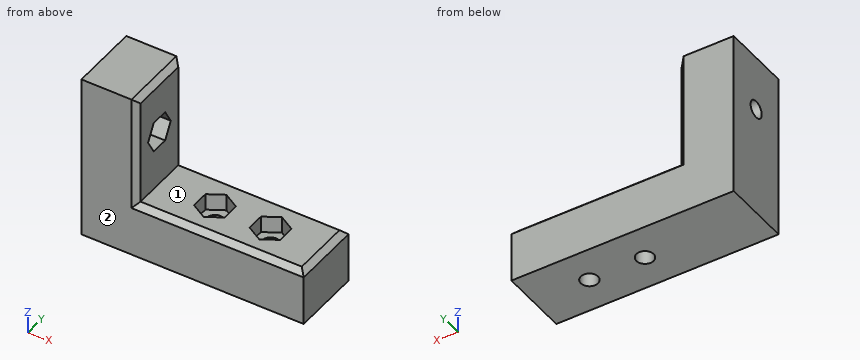
from build123d import *

# Parameters (mm, degrees)
F0_W     = 30
F0_H     = 12.5
F0_R     = 1.55
F1_DEPTH = 10
F0_W_2   = 10
F2_DEPTH = 30
F3_R     = 1.55
F4_DEPTH = 10
F5_SIZE  = 1
F7_DEPTH = 3
F9_DEPTH = 3


# Not quite as in the source:
# - a feature names something its author has since deleted; it is built from what else it names


with BuildPart() as f1:
    # F0 (on Top) → F1 (new body)
    with BuildSketch(Plane.XY):
        with Locations((25, 6.25)):
            Rectangle(F0_W, F0_H)
        with Locations((20, 6.25)):
            Circle(F0_R, mode=Mode.SUBTRACT)
        with Locations((30, 6.25)):
            Circle(F0_R, mode=Mode.SUBTRACT)
    extrude(amount=F1_DEPTH)

    # F0 (on Top) → F2 (join)
    with BuildSketch(Plane.XY):
        with Locations((5, 6.25)):
            Rectangle(F0_W_2, F0_H)
    extrude(amount=F2_DEPTH)

    # F3 (on face) → F4 (cut)
    with BuildSketch(Plane(origin=(0, 0, 0), x_dir=(0, -1, 0), z_dir=(-1, 0, 0))):
        with Locations((-6.25, 20)):
            Circle(F3_R)
    extrude(amount=-F4_DEPTH, mode=Mode.SUBTRACT)

    # F5
    f5_edges = [f1.edges().sort_by_distance(p)[0] for p in [
        (25, 0, 10),
        (40, 6.25, 10),
        (25, 12.5, 10),
        (10, 12.5, 20),
        (10, 6.25, 30),
        (10, 0, 20),
    ]]
    chamfer(f5_edges, length=F5_SIZE)

    # F6 (on face) → F7 (cut)
    with BuildSketch(Plane.XY.offset(10)):
        Polygon((22.75, 4.6622867597), (22.75, 7.8377132403), (20, 9.4254264805), (17.25, 7.8377132403), (17.25, 4.6622867597), (20, 3.0745735195), align=None)
        Polygon((32.75, 4.6622867597), (32.75, 7.8377132403), (30, 9.4254264805), (27.25, 7.8377132403), (27.25, 4.6622867597), (30, 3.0745735195), align=None)
    extrude(amount=-F7_DEPTH, mode=Mode.SUBTRACT)

    # F8 (on face) → F9 (cut)
    with BuildSketch(Plane.YZ.offset(10)):
        Polygon((4.6622867597, 17.25), (7.8377132403, 17.25), (9.4254264805, 20), (7.8377132403, 22.75), (4.6622867597, 22.75), (3.0745735195, 20), align=None)
    extrude(amount=-F9_DEPTH, mode=Mode.SUBTRACT)


solid = f1.part
Geometry check sheet. Reference: the model listing, model coordinates, mm. Face numbers are marked on the shaded views. A direction names the side the tool comes from. Give positions to 0.01 mm unless a question says otherwise; leave off trailing zeros. Order: outer loops, then holes, each group sorted by start corner. A loop starts at its lowest first (then second) coordinate and runs counter-clockwise, first axis right, second up.
1) Tool access check on the marked faces 1 and 2. Record the directions out of +Z, -Z, +X, -X, +Y, -Y that give a thin tool (end or side, any length) a straight path to the whole face; none if there is none.
Results are:
face 1: +Z, +X, +Y, -Y
face 2: +Z, -Z, +X, -X, -Y
2) Cross-section at B-B (z = 7.5). Record the boundary of the cut face in (x, y), then the cut area to 3 significant figures.
Results are:
outline: (0, 0) - (40, 0) - (40, 12.5) - (0, 12.5) - close; hole (17.25, 4.66) - (20, 3.07) - (22.75, 4.66) - (22.75, 7.84) - (20, 9.43) - (17.25, 7.84) - close; hole (27.25, 4.66) - (30, 3.07) - (32.75, 4.66) - (32.75, 7.84) - (30, 9.43) - (27.25, 7.84) - close
area: 448 mm2
3) Cross-section at D-D (x = 22). Record the boundary of the cut face in (y, z), then the cut area to 3 significant figures.
Results are:
outline: (0, 0) - (12.5, 0) - (12.5, 9) - (11.5, 10) - (8.27, 10) - (8.27, 7) - (4.23, 7) - (4.23, 10) - (1, 10) - (0, 9) - close
area: 112 mm2
4) Cross-section at C-C (z = 13). Record the boundary of the cut face in (x, y).
Results are:
outline: (0, 0) - (9, 0) - (10, 1) - (10, 11.5) - (9, 12.5) - (0, 12.5) - close
5) Gauge pin test, flat ends, axial feed: pin 1 (6 mm diameter, centred on x = 30.5, y = 5, fed in from +Z); pin 2 (6 mm diameter, centred on y = 4.5, z = 19, fed in from +X); pin 3 (1.6 mm diameter, centred on x = 21, y = 5.5, fed in from +Z). Record the tip position at first contact, or that the pin passes through.
Results are:
pin 1: stops at z = 10
pin 2: stops at x = 10
pin 3: stops at z = 7
6) Material ranges on probe 1 along X at (y, z) = (6.25, 4.5); probe 2 along Y at (x, z) = (20, 3.5); probe 3 along Z at (x, y) = (4, 6.25), recorded low to high.
Results are:
probe 1: x = 0 to 18.45, 21.55 to 28.45, 31.55 to 40
probe 2: y = 0 to 4.7, 7.8 to 12.5
probe 3: z = 0 to 18.45, 21.55 to 30
7) Cross-section at A-A (y = 6.25). Give the number of separate pieces and of enclosed holes in the cut face, then the cut area to 3 significant figures.
Results are:
separate pieces: 4
enclosed holes: 0
area: 484 mm2
